Model file for the job. Use its own axes, mm. Coordinates: 2 decimals unless noted, no trailing zeros. Loops run counter-clockwise (first coordinate to the right, second up) from the corner with the lowest first, then second, coordinate; pieces in that order, holes last. Notation, with made-up numbers: (73, -37.5) - (128, -37.5) arc R30 ccw to (128, -5.5) - close; hole circle Ø6 at (-23.75, -18.75). An arc over 180 degrees is marked (long way). Write each question's results on one line, items separated by ' | '. Start each with the question number.
```python
from build123d import *

# Parameters (mm, degrees)
SKETCH1_W           = 249.6
SKETCH1_H           = 350.4
SKETCH1_R           = 2.1
SKETCH1_R_2         = 2.5
SKETCH1_R_3         = 1.59
SKETCH1_R_4         = 12.5
SKETCH1_W_2         = 33
SKETCH1_H_2         = 90
BOSS_EXTRUDE1_DEPTH = 5
SKETCH12_W          = 249.6
SKETCH12_H          = 5
CUT_EXTRUDE2_DEPTH  = 83
CUT_EXTRUDE3_DEPTH  = 6


with BuildPart() as part:
    # Sketch1 → Boss-Extrude1 (new body)
    with BuildSketch(Plane.XY):
        with Locations((124.8, -175.2)):
            Rectangle(SKETCH1_W, SKETCH1_H)
        with Locations((104.3, -14)):
            Circle(SKETCH1_R, mode=Mode.SUBTRACT)
        with Locations((245.6, -124.5)):
            Circle(SKETCH1_R_2, mode=Mode.SUBTRACT)
        with Locations((245.6, -175.5)):
            Circle(SKETCH1_R_2, mode=Mode.SUBTRACT)
        with Locations((145.3, -14)):
            Circle(SKETCH1_R, mode=Mode.SUBTRACT)
        with Locations((179.16, -134.375)):
            Circle(SKETCH1_R_3, mode=Mode.SUBTRACT)
        with Locations((179.16, -165.625)):
            Circle(SKETCH1_R_3, mode=Mode.SUBTRACT)
        with Locations((124.8, -14)):
            Circle(SKETCH1_R_4, mode=Mode.SUBTRACT)
        with Locations((141.06, -134.375)):
            Circle(SKETCH1_R_3, mode=Mode.SUBTRACT)
        with Locations((153.76, -134.375)):
            Circle(SKETCH1_R_3, mode=Mode.SUBTRACT)
        with Locations((166.46, -134.375)):
            Circle(SKETCH1_R_3, mode=Mode.SUBTRACT)
        with Locations((141.06, -165.625)):
            Circle(SKETCH1_R_3, mode=Mode.SUBTRACT)
        with Locations((153.76, -165.625)):
            Circle(SKETCH1_R_3, mode=Mode.SUBTRACT)
        with Locations((166.46, -165.625)):
            Circle(SKETCH1_R_3, mode=Mode.SUBTRACT)
        with Locations((83.14, -165.625)):
            Circle(SKETCH1_R_3, mode=Mode.SUBTRACT)
        with Locations((95.84, -165.625)):
            Circle(SKETCH1_R_3, mode=Mode.SUBTRACT)
        with Locations((108.54, -165.625)):
            Circle(SKETCH1_R_3, mode=Mode.SUBTRACT)
        with Locations((83.14, -134.375)):
            Circle(SKETCH1_R_3, mode=Mode.SUBTRACT)
        with Locations((95.84, -134.375)):
            Circle(SKETCH1_R_3, mode=Mode.SUBTRACT)
        with Locations((108.54, -134.375)):
            Circle(SKETCH1_R_3, mode=Mode.SUBTRACT)
        with Locations((70.44, -165.625)):
            Circle(SKETCH1_R_3, mode=Mode.SUBTRACT)
        with Locations((70.44, -134.375)):
            Circle(SKETCH1_R_3, mode=Mode.SUBTRACT)
        with Locations((4, -175.5)):
            Circle(SKETCH1_R_2, mode=Mode.SUBTRACT)
        with Locations((4, -124.5)):
            Circle(SKETCH1_R_2, mode=Mode.SUBTRACT)
        with Locations((201.66, -150)):
            Rectangle(SKETCH1_W_2, SKETCH1_H_2, mode=Mode.SUBTRACT)
        with BuildLine():
            Line((145.8225, -134.375), (145.8225, -154.054634918))
            ThreePointArc((145.8225, -154.054634918), (147.41, -154.140223925), (148.9975, -154.054634918))
            Line((148.9975, -154.054634918), (148.9975, -134.375))
            ThreePointArc((148.9975, -134.375), (147.41, -132.7875), (145.8225, -134.375))
        make_face(mode=Mode.SUBTRACT)
        with BuildLine():
            Line((158.52, -134.375), (158.52, -154.054634918))
            ThreePointArc((158.52, -154.054634918), (160.11, -154.140492925), (161.7, -154.054634918))
            Line((161.7, -154.054634918), (161.7, -134.375))
            ThreePointArc((161.7, -134.375), (160.11, -132.785), (158.52, -134.375))
        make_face(mode=Mode.SUBTRACT)
        with BuildLine():
            Line((171.22, -134.375), (171.22, -154.054634918))
            ThreePointArc((171.22, -154.054634918), (172.81, -154.140492925), (174.4, -154.054634918))
            Line((174.4, -154.054634918), (174.4, -134.375))
            ThreePointArc((174.4, -134.375), (172.81, -132.785), (171.22, -134.375))
        make_face(mode=Mode.SUBTRACT)
        with BuildLine():
            Line((145.8225, -165.625), (145.8225, -185.304634918))
            ThreePointArc((145.8225, -185.304634918), (147.41, -185.390223925), (148.9975, -185.304634918))
            Line((148.9975, -185.304634918), (148.9975, -165.625))
            ThreePointArc((148.9975, -165.625), (147.41, -164.0375), (145.8225, -165.625))
        make_face(mode=Mode.SUBTRACT)
        with BuildLine():
            Line((158.52, -165.625), (158.52, -185.304634918))
            ThreePointArc((158.52, -185.304634918), (160.11, -185.390492925), (161.7, -185.304634918))
            Line((161.7, -185.304634918), (161.7, -165.625))
            ThreePointArc((161.7, -165.625), (160.11, -164.035), (158.52, -165.625))
        make_face(mode=Mode.SUBTRACT)
        with BuildLine():
            Line((171.22, -165.625), (171.22, -185.304634918))
            ThreePointArc((171.22, -185.304634918), (172.81, -185.390492925), (174.4, -185.304634918))
            Line((174.4, -185.304634918), (174.4, -165.625))
            ThreePointArc((174.4, -165.625), (172.81, -164.035), (171.22, -165.625))
        make_face(mode=Mode.SUBTRACT)
        with BuildLine():
            Line((103.7775, -134.375), (103.7775, -154.054634918))
            ThreePointArc((103.7775, -154.054634918), (102.19, -155.642134918), (100.6025, -154.054634918))
            Line((100.6025, -154.054634918), (100.6025, -134.375))
            ThreePointArc((100.6025, -134.375), (102.19, -132.7875), (103.7775, -134.375))
        make_face(mode=Mode.SUBTRACT)
        with BuildLine():
            Line((91.08, -134.375), (91.08, -154.054634918))
            ThreePointArc((91.08, -154.054634918), (89.49, -155.644634918), (87.9, -154.054634918))
            Line((87.9, -154.054634918), (87.9, -134.375))
            ThreePointArc((87.9, -134.375), (89.49, -132.785), (91.08, -134.375))
        make_face(mode=Mode.SUBTRACT)
        with BuildLine():
            Line((78.38, -134.375), (78.38, -154.054634918))
            ThreePointArc((78.38, -154.054634918), (76.79, -155.644634918), (75.2, -154.054634918))
            Line((75.2, -154.054634918), (75.2, -134.375))
            ThreePointArc((75.2, -134.375), (76.79, -132.785), (78.38, -134.375))
        make_face(mode=Mode.SUBTRACT)
        with BuildLine():
            Line((103.7775, -165.625), (103.7775, -185.304634918))
            ThreePointArc((103.7775, -185.304634918), (102.19, -186.892134918), (100.6025, -185.304634918))
            Line((100.6025, -185.304634918), (100.6025, -165.625))
            ThreePointArc((100.6025, -165.625), (102.19, -164.0375), (103.7775, -165.625))
        make_face(mode=Mode.SUBTRACT)
        with BuildLine():
            Line((91.08, -165.625), (91.08, -185.304634918))
            ThreePointArc((91.08, -185.304634918), (89.49, -186.894634918), (87.9, -185.304634918))
            Line((87.9, -185.304634918), (87.9, -165.625))
            ThreePointArc((87.9, -165.625), (89.49, -164.035), (91.08, -165.625))
        make_face(mode=Mode.SUBTRACT)
        with BuildLine():
            Line((78.38, -165.625), (78.38, -185.304634918))
            ThreePointArc((78.38, -185.304634918), (76.79, -186.894634918), (75.2, -185.304634918))
            Line((75.2, -185.304634918), (75.2, -165.625))
            ThreePointArc((75.2, -165.625), (76.79, -164.035), (78.38, -165.625))
        make_face(mode=Mode.SUBTRACT)
        with Locations((47.94, -150)):
            Rectangle(SKETCH1_W_2, SKETCH1_H_2, mode=Mode.SUBTRACT)
    extrude(amount=BOSS_EXTRUDE1_DEPTH)

    # Sketch12 → Cut-Extrude2 (cut)
    with BuildSketch(Plane.XZ.offset(350.4)):
        with Locations((124.8, 2.5)):
            Rectangle(SKETCH12_W, SKETCH12_H)
    extrude(amount=-CUT_EXTRUDE2_DEPTH, mode=Mode.SUBTRACT)

    # Sketch13 → Cut-Extrude3 (cut, through all)
    with BuildSketch(Plane.XY.offset(5)):
        with BuildLine():
            Line((43.402860001, -100), (0, -100))
            Line((0, -100), (0, 25))
            Line((0, 25), (43.402860001, 25))
            ThreePointArc((43.402860001, 25), (105.902860001, -37.5), (43.402860001, -100))
        make_face()
        with BuildLine():
            Line((206.197139999, 25), (249.6, 25))
            Line((249.6, 25), (249.6, -100))
            Line((249.6, -100), (206.197139999, -100))
            ThreePointArc((206.197139999, -100), (143.697139999, -37.5), (206.197139999, 25))
        make_face()
    extrude(amount=-CUT_EXTRUDE3_DEPTH, mode=Mode.SUBTRACT)


solid = part.part
```
Q1. Cut at B-B (z = 3.2). State how many separate pieces and enclosed holes the cut face has, and give its area (3 significant figures).
Q2. Pin check, flat tip, straight feed: pin 1 (1 mm diameter, centred on y = -77.5, z = 2.5, fed in from -X). Stop position of the tip, or through.
Q3. Cut at C-C (x = 25.5). List the corners of the cut face in (y, z).
Q4. Mould opens along Y. For faces 1 (the cylindrical face through (99.73, -64.58, 2.54)), 2 (the flat face through (123, -162, 5)) say: +Y half, -Y half, draft (parallel to the pull), parting line (faces both ways), or undercut.
Q5. Cut at D-D (y = -76). List the corners of the cut face in (x, z), and give its area (3 significant figures).
Q6. Drill centre lines: L1, parallel to X at y = -160, z = 3.05; L2, parallel to Y at x = 4, z = 2.3; L3, parallel to Y at x = 179.16, z = 1.55 (3 decimals). Where is each one in solid material? Low to high. Write a range as from..to.
Q7. Cut at A-A (x = 188.5). List the corners of the cut face in (y, z), and give its area (3 significant figures).
Check result:
1) separate pieces: 1 | enclosed holes: 37 | area: 40,100 mm²
2) pin 1: x = 91.01
3) outline: (-267.4, 0) - (-100, 0) - (-100, 5) - (-267.4, 5) - close
4) face 1: undercut | face 2: draft
5) outline: (92.64, 0) - (156.96, 0) - (156.96, 5) - (92.64, 5) - close | area: 322 mm²
6) L1: 0..31.44, 64.44..185.16, 218.16..249.6 | L2: -267.4..-178, -173..-127, -122..-100 | L3: -267.4..-167.215, -164.035..-135.965, -132.785..-93.849
7) outline: (-267.4, 0) - (-195, 0) - (-195, 5) - (-267.4, 5) - close; (-105, 0) - (-97.44, 0) - (-97.44, 5) - (-105, 5) - close | area: 400 mm²
